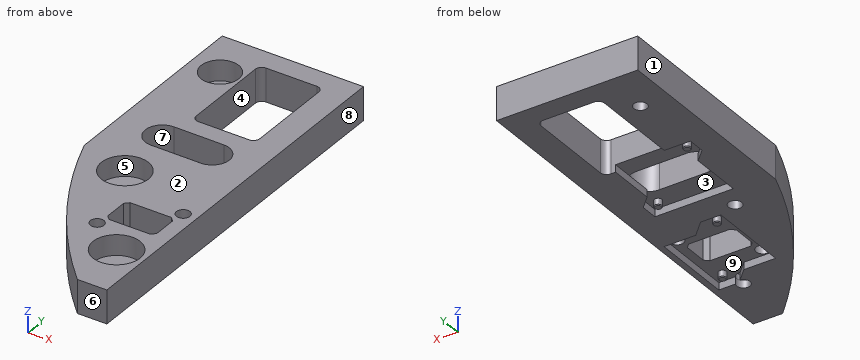
```python
from build123d import *

# Parameters (mm, degrees)
SKETCH1_R           = 2.15265
BOSS_EXTRUDE1_DEPTH = 2.3495
SKETCH2_R           = 2.15265
SKETCH2_R_2         = 2.195581339
SKETCH2_W           = 15.875
SKETCH2_H           = 10.16
BOSS_EXTRUDE2_DEPTH = 8.4455
SKETCH3_R           = 1.22555
BOSS_EXTRUDE3_DEPTH = 2.159
CHAMFER1_SIZE       = 0.254
CHAMFER2_SIZE       = 1.27
SKETCH5_R           = 7.62
SKETCH5_R_2         = 6.096
CUT_EXTRUDE1_DEPTH  = 6.604


with BuildPart() as part:
    # Sketch1 → Boss-Extrude1 (new body)
    with BuildSketch(Plane.XY):
        with BuildLine():
            Line((0, -17.78), (-45.72, -17.78))
            Line((-45.72, -17.78), (-45.72, -84.1375))
            ThreePointArc((-45.72, -84.1375), (-30.833523511, -114.746148224), (-9.525, -141.2875))
            Line((-9.525, -141.2875), (0, -141.2875))
            Line((0, -141.2875), (0, -17.78))
        make_face()
        with Locations((-36.1315, -33.274)):
            Circle(SKETCH1_R, mode=Mode.SUBTRACT)
        with Locations((-29.5275, -88.7095)):
            Circle(SKETCH1_R, mode=Mode.SUBTRACT)
        with BuildLine():
            Line((-1.89756812, -121.923613785), (-1.89756812, -95.571113785))
            Line((-1.89756812, -95.571113785), (-12.166516896, -95.571113785))
            Line((-12.166516896, -95.571113785), (-16.929016896, -90.808613785))
            Line((-16.929016896, -90.808613785), (-23.48756812, -90.808613785))
            Line((-23.48756812, -90.808613785), (-23.48756812, -117.161113785))
            Line((-23.48756812, -117.161113785), (-13.218619344, -117.161113785))
            Line((-13.218619344, -117.161113785), (-9.502774703, -120.876958426))
            ThreePointArc((-9.502774703, -120.876958426), (-10.060883947, -124.947120561), (-7.279497151, -121.923613785))
            Line((-7.279497151, -121.923613785), (-1.89756812, -121.923613785))
        make_face(mode=Mode.SUBTRACT)
        with BuildLine():
            Line((-33.655, -81.7245), (-8.255, -81.7245))
            Line((-8.255, -81.7245), (-8.255, -76.118448776))
            Line((-8.255, -76.118448776), (-12.065, -72.308448776))
            Line((-12.065, -72.308448776), (-12.065, -57.1627))
            Line((-12.065, -57.1627), (-10.4902, -57.1627))
            ThreePointArc((-10.4902, -57.1627), (-9.053359021, -56.567540979), (-8.4582, -55.1307))
            Line((-8.4582, -55.1307), (-8.4582, -26.6573))
            ThreePointArc((-8.4582, -26.6573), (-9.053359021, -25.220459021), (-10.4902, -24.6253))
            Line((-10.4902, -24.6253), (-26.9748, -24.6253))
            ThreePointArc((-26.9748, -24.6253), (-28.411640979, -25.220459021), (-29.0068, -26.6573))
            Line((-29.0068, -26.6573), (-29.0068, -55.372))
            Line((-29.0068, -55.372), (-37.465, -55.372))
            Line((-37.465, -55.372), (-37.465, -60.978051224))
            Line((-37.465, -60.978051224), (-33.655, -64.788051224))
            Line((-33.655, -64.788051224), (-33.655, -81.7245))
        make_face(mode=Mode.SUBTRACT)
    extrude(amount=BOSS_EXTRUDE1_DEPTH)

    # Sketch2 → Boss-Extrude2 (add)
    with BuildSketch(Plane.XY.offset(2.3495)):
        with BuildLine():
            Line((-9.525, -141.2875), (0, -141.2875))
            Line((0, -141.2875), (0, -17.78))
            Line((0, -17.78), (-45.72, -17.78))
            Line((-45.72, -17.78), (-45.72, -84.1375))
            ThreePointArc((-45.72, -84.1375), (-30.833523511, -114.746148224), (-9.525, -141.2875))
        make_face()
        with Locations((-9.144, -122.9995)):
            Circle(SKETCH2_R, mode=Mode.SUBTRACT)
        with Locations((-29.5275, -88.7095)):
            Circle(SKETCH2_R, mode=Mode.SUBTRACT)
        with Locations((-21.016048243, -114.689593907)):
            Circle(SKETCH2_R_2, mode=Mode.SUBTRACT)
        with Locations((-4.369087998, -98.042633662)):
            Circle(SKETCH2_R_2, mode=Mode.SUBTRACT)
        with Locations((-36.1315, -33.274)):
            Circle(SKETCH2_R, mode=Mode.SUBTRACT)
        with Locations((-12.69256812, -106.366113785)):
            Rectangle(SKETCH2_W, SKETCH2_H, mode=Mode.SUBTRACT)
        with BuildLine():
            Line((-14.798016067, -74.184431866), (-30.952016067, -74.104431866))
            ThreePointArc((-30.952016067, -74.104431866), (-36.480681866, -68.520733933), (-30.896983933, -62.992068134))
            Line((-30.896983933, -62.992068134), (-14.742983933, -63.072068134))
            ThreePointArc((-14.742983933, -63.072068134), (-9.214318134, -68.655766067), (-14.798016067, -74.184431866))
        make_face(mode=Mode.SUBTRACT)
        with BuildLine():
            Line((-8.4582, -55.1307), (-8.4582, -26.6573))
            ThreePointArc((-8.4582, -26.6573), (-9.053359021, -25.220459021), (-10.4902, -24.6253))
            Line((-10.4902, -24.6253), (-26.9748, -24.6253))
            ThreePointArc((-26.9748, -24.6253), (-28.411640979, -25.220459021), (-29.0068, -26.6573))
            Line((-29.0068, -26.6573), (-29.0068, -55.1307))
            ThreePointArc((-29.0068, -55.1307), (-28.411640979, -56.567540979), (-26.9748, -57.1627))
            Line((-26.9748, -57.1627), (-10.4902, -57.1627))
            ThreePointArc((-10.4902, -57.1627), (-9.053359021, -56.567540979), (-8.4582, -55.1307))
        make_face(mode=Mode.SUBTRACT)
    extrude(amount=BOSS_EXTRUDE2_DEPTH)

    # Sketch3 → Boss-Extrude3 (add)
    with BuildSketch(Plane(origin=(0, 0, 2.3495), x_dir=(-1, 0, 0), z_dir=(0, 0, -1))):
        with Locations((34.29, -58.547)):
            Circle(SKETCH3_R)
        with Locations((11.43, -78.5495)):
            Circle(SKETCH3_R)
        with Locations((5.54881812, -118.272363785)):
            Circle(SKETCH3_R)
        with Locations((19.83631812, -94.459863785)):
            Circle(SKETCH3_R)
    extrude(amount=BOSS_EXTRUDE3_DEPTH)

    # Chamfer1
    chamfer1_edges = [part.edges().sort_by_distance(p)[0] for p in [
        (-33.06445, -58.547, 0.1905),
        (-10.20445, -78.5495, 0.1905),
        (-4.32326812, -118.272363785, 0.1905),
        (-18.61076812, -94.459863785, 0.1905),
    ]]
    chamfer(chamfer1_edges, length=CHAMFER1_SIZE)

    # Chamfer2
    chamfer2_edges = [part.edges().sort_by_distance(p)[0] for p in [
        (-20.63006812, -111.446113785, 6.57225),
        (-4.75506812, -111.446113785, 6.57225),
        (-4.75506812, -101.286113785, 6.57225),
        (-20.63006812, -101.286113785, 6.57225),
    ]]
    chamfer(chamfer2_edges, length=CHAMFER2_SIZE)

    # Sketch5 → Cut-Extrude1 (cut)
    with BuildSketch(Plane.XY.offset(10.795)):
        with Locations((-9.144, -122.9995)):
            Circle(SKETCH5_R)
        with Locations((-29.5275, -88.7095)):
            Circle(SKETCH5_R)
        with Locations((-36.068, -33.2105)):
            Circle(SKETCH5_R_2)
    extrude(amount=-CUT_EXTRUDE1_DEPTH, mode=Mode.SUBTRACT)


solid = part.part
```
Verification items for the finished model (mm, model axes). Face numbers are marked on the shaded views. A direction names the side the tool comes from. Round coordinates to 2 decimals unless told otherwise and drop trailing zeros. Put each result on its own line as item: value. Start each with the question number.
(1) Draft check along Y on the marked faces 6, 7, 8 and 9. Enter one of: +Y half, -Y half, draft (parallel to the pull), parting line (faces both ways), or undercut.
(2) Depth check by flat-ended pin: pin 1 Ø2.5 at (x, z) = (-19.5, 1.5) entering from -Y; pin 2 Ø6 at (y, z) = (-98.5, 3.5) entering from -X; pin 3 Ø4 at (x, z) = (-21.5, 6.5) entering from -Y. Enter the tip coordinate at first touch or a pass-through.
(3) Section check A-A (z = 9.25). State how many separate pieces and enclosed holes the cut face has, then the cut area to 3 significant figures.
(4) Material ranges on line 1 along Y through (x, z) = (-5, 9.25); line 2 along Y through (x, z) = (-35.5, 4.5); line 3 along Y through (x, z) = (-11, 7.5), recorded low to high.
(5) Tool access check on the marked faces 1, 2, 3, 4 and 5. Record the directions out of +Z, -Z, +X, -X, +Y, -Y that give a thin tool (end or side, any length) a straight path to the whole face; none if there is none.
Completed:
1. face 6: -Y half
1. face 7: undercut
1. face 8: draft
1. face 9: undercut
2. pin 1: stops at y = -131.85
2. pin 2: stops at x = -41.17
2. pin 3: stops at y = -130.36
3. separate pieces: 1
3. enclosed holes: 8
3. area: 3,170 mm2
4. line 1: y = -141.29 to -129.39, -116.6 to -110.42, -102.31 to -100.15, -95.94 to -17.78
4. line 2: y = -106.86 to -93.44, -83.98 to -71.7, -65.4 to -39.28, -27.14 to -17.78
4. line 3: y = -139.8 to -130.39, -115.61 to -111.45, -101.29 to -72.71, -64.55 to -57.16, -24.63 to -17.78
5. face 1: +Z, -Z, -X, +Y, -Y
5. face 2: +Z, +X, -X, +Y, -Y
5. face 3: -Z
5. face 4: +Z, -Z
5. face 5: +Z
